Source: CAD feature listing. Evaluate the final solid. Frame: model axes, mm. Give positions to 0.01 mm unless a question says otherwise; leave off trailing zeros. Write each loop counter-clockwise with the first axis right and the second up, starting at its lowest first coordinate (ties: lowest second). Pieces come first, ordered by that corner, then holes. Notation, with made-up numbers: (61.5, -19) -> (118.5, -19) arc R19 cw to (118.5, 4) -> close; hole circle Ø4 at (-33.75, 42). An arc over 180 degrees is marked (long way). Write item = value, one per line.
from build123d import *

# Parameters (mm, degrees)
BOSS_EXTRUDE1_DEPTH = 4
SKETCH2_R           = 11
CUT_EXTRUDE1_DEPTH  = 135.595690867


with BuildPart() as part:
    # Sketch1 → Boss-Extrude1 (new body)
    with BuildSketch(Plane.XY):
        Polygon((0, 0), (90, 0), (90, 100), (70, 100), (0, 50), align=None)
    extrude(amount=BOSS_EXTRUDE1_DEPTH)

    # Sketch2 → Cut-Extrude1 (cut, through all)
    with BuildSketch(Plane(origin=(0, 0, 0), x_dir=(-1, 0, 0), z_dir=(0, 0, -1))):
        with Locations((-21.867101934, 12.5)):
            Circle(SKETCH2_R)
    extrude(amount=-CUT_EXTRUDE1_DEPTH, mode=Mode.SUBTRACT)


solid = part.part
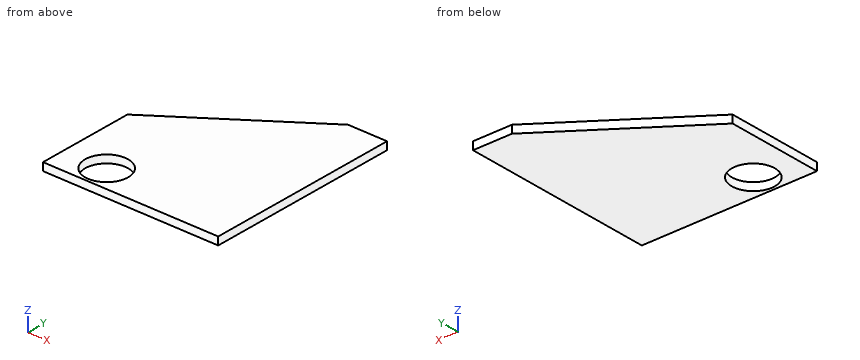
(1) First-contact query: pin 1 (1.5 mm diameter, centred on x = 28, z = 3, fed in from +Y). Flat tip, straight axial feed; report the tip coordinate or a pass-through.
Values follow:
pin_1 = 70.54
(2) Material intervals for line 1 (Y direction, x = 42.5, z = 1.35); line 2 (Y direction, x = 18.5, z = 3.8); line 3 (Y direction, x = 39, z = 0.4), sorted ascending.
Values follow:
line_1 = 0 to 80.36
line_2 = 0 to 2.03, 22.97 to 63.21
line_3 = 0 to 77.86
(3) Section query B-B (z = 2.5). Return loops of the section in (x, y), plus the area to 3 significant figures.
Values follow:
outline = (0, 0) -> (90, 0) -> (90, 100) -> (70, 100) -> (0, 50) -> close; hole circle Ø22 at (21.87, 12.5)
area = 6,870 mm2
(4) Section query D-D (y = 82). Return loops of the section in (x, z).
Values follow:
outline = (44.8, 0) -> (90, 0) -> (90, 4) -> (44.8, 4) -> close
(5) Section query C-C (x = 8.5). Return loops of the section in (y, z), plus the area to 3 significant figures.
Values follow:
outline = (0, 0) -> (56.07, 0) -> (56.07, 4) -> (0, 4) -> close
area = 224 mm2
(6) Section query A-A (y = 12.5). Return loops of the section in (x, z), plus the area to 3 significant figures.
Values follow:
outline = (0, 0) -> (10.87, 0) -> (10.87, 4) -> (0, 4) -> close; (32.87, 0) -> (90, 0) -> (90, 4) -> (32.87, 4) -> close
area = 272 mm2
